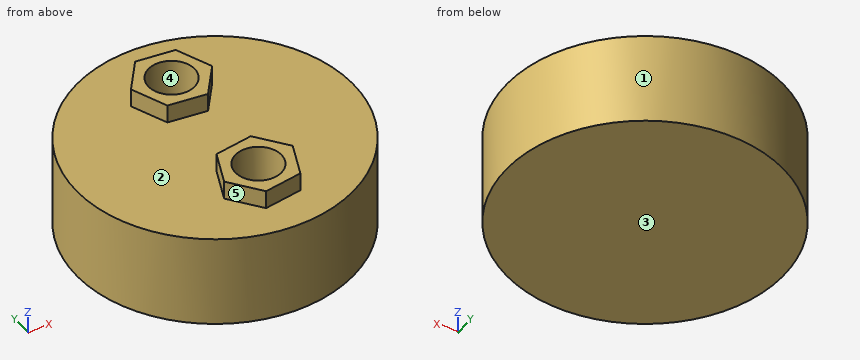
from build123d import *

# Parameters (mm, degrees)
IZIM1_R                     = 15
Y_KSEKLIK_EKSTR_ZYON1_DEPTH = 10
IZIM2_R                     = 2.5
KES_EKSTR_ZYON1_DEPTH       = 5
Y_KSEKLIK_EKSTR_ZYON3_START = 2
IZIM3_R                     = 2.5
Y_KSEKLIK_EKSTR_ZYON3_DEPTH = 2


with BuildPart() as part:
    # Çizim1 → Yükseklik-Ekstrüzyon1 (new body)
    with BuildSketch(Plane.XY):
        Circle(IZIM1_R)
    extrude(amount=Y_KSEKLIK_EKSTR_ZYON1_DEPTH)

    # Çizim2 → Kes-Ekstrüzyon1 (cut)
    with BuildSketch(Plane.XY.offset(10)):
        with Locations((0, 7.5)):
            Circle(IZIM2_R)
        with Locations((0, -7.5)):
            Circle(IZIM2_R)
    extrude(amount=-KES_EKSTR_ZYON1_DEPTH, mode=Mode.SUBTRACT)

    # Çizim3 → Yükseklik-Ekstrüzyon3 (add)
    # profile 1 of 2: a face of its own
    with BuildSketch(Plane.XY.offset(10).offset(Y_KSEKLIK_EKSTR_ZYON3_START)):
        Polygon((-4.083040029, 8.04725253), (-2.515454607, 4.237609875), (1.567585421, 3.690357346), (4.083040029, 6.95274747), (2.515454607, 10.762390125), (-1.567585421, 11.309642654), align=None)
        with Locations((0, 7.5)):
            Circle(IZIM3_R, mode=Mode.SUBTRACT)
    # profile 2 of 2: a face of its own
    with BuildSketch(Plane.XY.offset(10).offset(Y_KSEKLIK_EKSTR_ZYON3_START)):
        Polygon((1.567585421, -3.690357346), (4.083040029, -6.95274747), (2.515454607, -10.762390125), (-1.567585421, -11.309642654), (-4.083040029, -8.04725253), (-2.515454607, -4.237609875), align=None)
        with Locations((0, -7.5)):
            Circle(IZIM3_R, mode=Mode.SUBTRACT)
    extrude(amount=-Y_KSEKLIK_EKSTR_ZYON3_DEPTH)


solid = part.part
Source: CAD feature listing. Evaluate the final solid. Frame: model axes, mm. Face numbers are marked on the shaded views. A direction names the side the tool comes from. Give positions to 0.01 mm unless a question says otherwise; leave off trailing zeros. Write each loop counter-clockwise with the first axis right and the second up, starting at its lowest first coordinate (ties: lowest second). Pieces come first, ordered by that corner, then holes. Notation, with made-up numbers: M -10.75,19.5 L 11.25,19.5 A28 ccw 11.25,40.5 Z; hole C 32,79 d9. An arc over 180 degrees is marked long. Return JSON: item names as keys, results as strings. Group by question number.
1) Set-up query: the marked faces 4 and 5. Return all of +Z, -Z, +X, -X, +Y, -Y with unobstructed straight access to the full face (end or side cutting, diameter ignored); none if empty.
2) Ray query, L1, parallel to Y at x = 0, z = 6.5; L2, parallel to Z at x = 4.75, y = 2; L3, parallel to X at y = 5.25, z = 7.5. Return the intervals inside material, ascending.
3) Cut plane C-C, the plane z = 6.25. Output: boundary loops of the cut face in (x, y).
4) Cut plane D-D, the plane x = 0. Output: boundary loops of the cut face in (y, z).
5) First-contact query: pin 1 Ø9 at (x, y) = (-2, -7.5) entering from +Z; pin 2 Ø1.5 at (y, z) = (-4, 9.5) entering from +X; pin 3 Ø6 at (y, z) = (-4, 7.5) entering from -X; pin 4 Ø3 at (y, z) = (-11, 5) entering from -X. Flat tips, straight axial feed; report the tip coordinate or a pass-through.
6) Draft query along Y for the marked faces 1, 2 and 3. Return one class per face: released by +Y, released by -Y, zero draft, split by the parting line, or undercut.
7) Cut plane A-A, the plane z = 11. Output: boundary loops of the cut face in (x, y), then the cut area to 3 significant figures.
8) Cut plane B-B, the plane y = -7.5. Output: boundary loops of the cut face in (x, z), then the cut area to 3 significant figures.
Data:
{
 "1": {"face 4": "+Z", "face 5": "+Z, -X, -Y"},
 "2": {"L1": "y = -15 to -10, -5 to 5, 10 to 15", "L2": "z = 0 to 10", "L3": "x = -14.05 to -1.09, 1.09 to 14.05"},
 "3": {"outline": "C 0,0 d30; hole C 0,-7.5 d5; hole C 0,7.5 d5"},
 "4": {"outline": "M -15,0 L 15,0 L 15,10 L 11.1,10 L 11.1,12 L 10,12 L 10,5 L 5,5 L 5,12 L 3.9,12 L 3.9,10 L -3.9,10 L -3.9,12 L -5,12 L -5,5 L -10,5 L -10,12 L -11.1,12 L -11.1,10 L -15,10 Z"},
 "5": {"pin 1": "stops at z = 12", "pin 2": "stops at x = 14.64", "pin 3": "stops at x = -14.97", "pin 4": "stops at x = -11.61"},
 "6": {"face 1": "split by the parting line", "face 2": "undercut", "face 3": "zero draft"},
 "7": {"outline": "M -4.08,-8.05 L -1.57,-11.31 L 2.52,-10.76 L 4.08,-6.95 L 1.57,-3.69 L -2.52,-4.24 Z; M -4.08,8.05 L -2.52,4.24 L 1.57,3.69 L 4.08,6.95 L 2.52,10.76 L -1.57,11.31 Z; hole C 0,-7.5 d5; hole C 0,7.5 d5", "area": "48.9 mm²"},
 "8": {"outline": "M -12.99,0 L 12.99,0 L 12.99,10 L 3.86,10 L 3.86,12 L 2.5,12 L 2.5,5 L -2.5,5 L -2.5,12 L -3.86,12 L -3.86,10 L -12.99,10 Z", "area": "240 mm²"}
}
